from build123d import *

# Parameters (mm, degrees)
F0_R     = 110
F1_DEPTH = 20
F2_R     = 5.5
F2_R_2   = 10
F3_DEPTH = 25
F4_R     = 5
F5_DEPTH = 25


with BuildPart() as f1:
    # F0 (on Front) → F1 (new body)
    with BuildSketch(Plane.XZ):
        Circle(F0_R)
    extrude(amount=F1_DEPTH)

    # F2 (on face) → F3 (cut)
    with BuildSketch(Plane.XZ.offset(20)):
        with Locations((84.852814, 0)):
            Circle(F2_R)
        with Locations((60, 60)):
            Circle(F2_R)
        with Locations((0, 84.852814)):
            Circle(F2_R)
        with Locations((-60, 60)):
            Circle(F2_R)
        with Locations((-84.852814, 0)):
            Circle(F2_R)
        with Locations((-60, -60)):
            Circle(F2_R)
        with Locations((0, -84.852814)):
            Circle(F2_R)
        with Locations((60, -60)):
            Circle(F2_R)
        Circle(F2_R_2)
        with Locations((52.262519, 21.647844)):
            Circle(F2_R)
        with Locations((52.262519, -21.647844)):
            Circle(F2_R)
        with Locations((21.647844, -52.262519)):
            Circle(F2_R)
        with Locations((-21.647844, -52.262519)):
            Circle(F2_R)
        with Locations((-52.262519, -21.647844)):
            Circle(F2_R)
        with Locations((-52.262519, 21.647844)):
            Circle(F2_R)
        with Locations((-21.647844, 52.262519)):
            Circle(F2_R)
        with Locations((21.647844, 52.262519)):
            Circle(F2_R)
    extrude(amount=-F3_DEPTH, mode=Mode.SUBTRACT)

    # F4 (on face) → F5 (cut)
    with BuildSketch(Plane.XZ.offset(20)):
        with Locations((25, 0)):
            Circle(F4_R)
        with Locations((12.5, 21.650635)):
            Circle(F4_R)
        with Locations((-12.5, 21.650635)):
            Circle(F4_R)
        with Locations((-25, 0)):
            Circle(F4_R)
        with Locations((-12.5, -21.650635)):
            Circle(F4_R)
        with Locations((12.5, -21.650635)):
            Circle(F4_R)
    extrude(amount=-F5_DEPTH, mode=Mode.SUBTRACT)


solid = f1.part
Design review of the part built by this model. Coordinates are the model's own, in mm. Coordinates: 2 decimals unless noted, no trailing zeros. Order: outer loops, then holes, each group sorted by start corner. A loop starts at its lowest first (then second) coordinate and runs counter-clockwise, first axis right, second up.
Item 1: Take a section at B-B, the plane x = 0. Write out the cut boundary in (y, z).
Item 2: Take a section at A-A, the plane z = 0. Write out the cut boundary in (x, y).
Item 3: For line 1 (Z direction, x = 0, y = -11.75); line 2 (X direction, y = -2, z = -53); line 3 (X direction, y = -5, z = -17.5), list the stretches that pass through material, from the lowest coordinate up.
Item 4: For pin 1 Ø4 at (y, z) = (-14.5, -24) entering from -X; pin 2 Ø3 at (x, y) = (-40, -18) entering from -Z; pin 3 Ø2 at (y, z) = (-2.5, -54) entering from -X, all flat-tipped, find the tip position at first contact; note any pin that passes through.
Item 5: Take a section at C-C, the plane y = -7.25. Count the separate pieces of the cut face and the enclosed holes in it, then the cut area to 3 significant figures.
Item 6: The part is to be moulded in two halves that separate along X. For faces 1 (the flat face through (-2, 0, -23)), 2 (the cylindrical face through (-23.846, -9.86, -107.384)), 3 (the cylindrical face through (20.93, -10.14, -46.81)), say which applies: pulls with the +X half, pulls with the -X half, needs draft (parallel to the pull), parting line crosses it, or undercut.
Item 7: Take a section at D-D, the plane x = 73.5. Write out the cut boundary in (y, z).
The answers:
1. outline: (-20, -110) - (0, -110) - (0, -90.35) - (-20, -90.35) - close; (-20, -79.35) - (0, -79.35) - (0, -10) - (-20, -10) - close; (-20, 10) - (0, 10) - (0, 79.35) - (-20, 79.35) - close; (-20, 90.35) - (0, 90.35) - (0, 110) - (-20, 110) - close
2. outline: (-110, -20) - (-90.35, -20) - (-90.35, 0) - (-110, 0) - close; (-79.35, -20) - (-30, -20) - (-30, 0) - (-79.35, 0) - close; (-20, -20) - (-10, -20) - (-10, 0) - (-20, 0) - close; (10, -20) - (20, -20) - (20, 0) - (10, 0) - close; (30, -20) - (79.35, -20) - (79.35, 0) - (30, 0) - close; (90.35, -20) - (110, -20) - (110, 0) - (90.35, 0) - close
3. line 1: z = -110 to -90.35, -79.35 to -10, 10 to 79.35, 90.35 to 110
3. line 2: x = -96.39 to -27.1, -16.2 to 16.2, 27.1 to 96.39
3. line 3: x = -108.6 to -55.87, -48.65 to -15.29, -9.71 to 9.71, 15.29 to 48.65, 55.87 to 108.6
4. pin 1: stops at x = -107.78
4. pin 2: stops at z = -103.04
4. pin 3: stops at x = -96.39
5. separate pieces: 1
5. enclosed holes: 23
5. area: 35,700 mm2
6. face 1: needs draft
6. face 2: parting line crosses it
6. face 3: undercut
7. outline: (-20, -81.84) - (0, -81.84) - (0, 81.84) - (-20, 81.84) - close
